Could you check a few things on this model? Use its own coordinates, in mm. A direction names the side the tool comes from. Round coordinates to 2 decimals unless told otherwise and drop trailing zeros. Write each loop counter-clockwise with the first axis right and the second up, starting at its lowest first coordinate (ties: lowest second). Pieces come first, ordered by that corner, then holes. Notation, with made-up numbers: (36, 33.25) -> (48, 33.25) arc R15 ccw to (48, 53.25) -> close; hole circle Ø4 at (65, 63.25). An arc over 180 degrees is marked (long way). Answer in a Markdown table with one row per item.
from build123d import *

# Parameters (mm, degrees)
SKETCH1_W           = 12.7
SKETCH1_H           = 12.7
SKETCH1_R           = 3.9878
BOSS_EXTRUDE1_DEPTH = 12.7
FILLET1_SIZE        = 7.9756
CUT_EXTRUDE2_DEPTH  = 6.35
SKETCH1_3_R         = 3.9878
CUT_EXTRUDE3_DEPTH  = 24.759524566


with BuildPart() as part:
    # Sketch1 → Boss-Extrude1 (new body)
    # profile 1 of 3: a face of its own
    with BuildSketch(Plane.XY):
        with Locations((0, 12.7)):
            Rectangle(SKETCH1_W, SKETCH1_H)
    # profile 2 of 3: a face of its own
    with BuildSketch(Plane.XY):
        Rectangle(SKETCH1_W, SKETCH1_H)
        Circle(SKETCH1_R, mode=Mode.SUBTRACT)
    # profile 3 of 3: a face of its own
    with BuildSketch(Plane.XY):
        Circle(SKETCH1_R)
    extrude(amount=-BOSS_EXTRUDE1_DEPTH)

    # Fillet1
    # a fillet whose section is not a circle: 7.9756 mm, written as the material it takes off along each edge
    with BuildSketch(Plane(origin=(-6.35, -6.35, 19.939), x_dir=(1, 0, 0), z_dir=(0, 0, -1)), Plane(origin=(6.35, -6.35, 19.939), x_dir=(0, 1, 0), z_dir=(0, 0, -1))) as fillet1_piece_1:
        with BuildLine():
            add(Edge.make_bspline([(FILLET1_SIZE, 0), (FILLET1_SIZE * 0.831801948466, 0), (FILLET1_SIZE * 0.663603896932, 0), (FILLET1_SIZE * 0.292893218813, -FILLET1_SIZE * 0.0716919198361), (FILLET1_SIZE * 0.0716919198361, -FILLET1_SIZE * 0.292893218813), (0, -FILLET1_SIZE * 0.663603896932), (0, -FILLET1_SIZE * 0.831801948466), (0, -FILLET1_SIZE)], knots=[0, 0, 0, 0, 0, 0, 0.5, 0.5, 1, 1, 1, 1, 1, 1], degree=5))
            Line((0, -FILLET1_SIZE), (0, 0))
            Line((0, 0), (FILLET1_SIZE, 0))
        make_face()
    extrude(amount=52.578, mode=Mode.SUBTRACT)

    # Sketch3 → Cut-Extrude2 (cut)
    with BuildSketch(Plane(origin=(0, 19.05, 0), x_dir=(1, 0, 0), z_dir=(0, 1, 0))):
        with BuildLine():
            ThreePointArc((1.9939, 8.89), (1.409900211, 10.299900211), (0, 10.8839))
            Line((0, 10.8839), (0, 8.89))
            Line((0, 8.89), (1.9939, 8.89))
        make_face()
        with BuildLine():
            Line((0, 8.89), (0, 10.8839))
            ThreePointArc((0, 10.8839), (-1.409900211, 10.299900211), (-1.9939, 8.89))
            Line((-1.9939, 8.89), (0, 8.89))
        make_face()
        with BuildLine():
            Line((1.9939, 8.89), (0, 8.89))
            Line((0, 8.89), (0, 6.8961))
            ThreePointArc((0, 6.8961), (1.409900211, 7.480099789), (1.9939, 8.89))
        make_face()
        with BuildLine():
            Line((0, 6.8961), (0, 8.89))
            Line((0, 8.89), (-1.9939, 8.89))
            ThreePointArc((-1.9939, 8.89), (-1.409900211, 7.480099789), (0, 6.8961))
        make_face()
        with BuildLine():
            ThreePointArc((1.9939, 3.81), (1.409900211, 5.219900211), (0, 5.8039))
            Line((0, 5.8039), (0, 3.81))
            Line((0, 3.81), (1.9939, 3.81))
        make_face()
        with BuildLine():
            Line((0, 3.81), (0, 5.8039))
            ThreePointArc((0, 5.8039), (-1.409900211, 5.219900211), (-1.9939, 3.81))
            Line((-1.9939, 3.81), (0, 3.81))
        make_face()
        with BuildLine():
            ThreePointArc((0, 1.8161), (1.409900211, 2.400099789), (1.9939, 3.81))
            Line((1.9939, 3.81), (0, 3.81))
            Line((0, 3.81), (0, 1.8161))
        make_face()
        with BuildLine():
            Line((0, 3.81), (-1.9939, 3.81))
            ThreePointArc((-1.9939, 3.81), (-1.409900211, 2.400099789), (0, 1.8161))
            Line((0, 1.8161), (0, 3.81))
        make_face()
    extrude(amount=-CUT_EXTRUDE2_DEPTH, mode=Mode.SUBTRACT)

    # Sketch1<3> → Cut-Extrude3 (cut, through all)
    with BuildSketch(Plane.XY):
        Circle(SKETCH1_3_R)
    extrude(amount=-CUT_EXTRUDE3_DEPTH, mode=Mode.SUBTRACT)


solid = part.part
1) For pin 1 (6.5 mm diameter, centred on x = 0, y = 0, fed in from -Z); pin 2 (3 mm diameter, centred on y = -3, z = -3.5, fed in from +X), each with a flat end and sliding along its axis, tell me the tip position at first contact or that it passes through.
Findings:
| item | result |
|---|---|
| pin 1 | passes through |
| pin 2 | stops at x = 6.12 |
2) Thinking about a two-plate mould opening in Z: for faces 3 (the face through (0, 12.7, -4)), 4 (the face through (3.804, 1.198, -6.261)), 5 (the face through (0, 9, -12.7)), which applies, +Z half, -Z half, draft (parallel to the pull), parting line (faces both ways), or undercut?
Findings:
| item | result |
|---|---|
| face 3 | undercut |
| face 4 | draft |
| face 5 | -Z half |
3) For faces 1 (the face through (-6.35, 10, -6)), 2 (the face through (0, 12.7, -9)), which set-ups out of +Z, -Z, +X, -X, +Y, -Y let a thin tool reach every point of the face, with its end or its side?
Findings:
| item | result |
|---|---|
| face 1 | +Z, -Z, -X, +Y, -Y |
| face 2 | +Y |
4) Please list where these lines run through material, in increasing order: line 1 (Y direction, x = 0, z = -3); line 2 (Y direction, x = 0, z = -6.5); line 3 (X direction, y = 16, z = -5.5).
Findings:
| item | result |
|---|---|
| line 1 | y = -6.31 to -3.99, 3.99 to 12.7 |
| line 2 | y = -6.31 to -3.99, 3.99 to 19.05 |
| line 3 | x = -6.35 to -1.06, 1.06 to 6.35 |
5) Imagine slicing it at A-A, the plane y = 13.5. Please give me the cut outline in (x, z), plus the area to 3 significant figures.
Findings:
| item | result |
|---|---|
| outline | (-6.35, -12.7) -> (6.35, -12.7) -> (6.35, 0) -> (-6.35, 0) -> close; hole circle Ø3.99 at (0, -8.89); hole circle Ø3.99 at (0, -3.81) |
| area | 136 mm^2 |
